Check sheet for the drawn part. Datum: minimum x, y, z corner. Units: mm. A direction names the side the tool comes from. Give positions to 0.01 mm unless a question says otherwise; leave off trailing zeros. Order: outer loops, then holes, each group sorted by start corner. A loop starts at its lowest first (then second) coordinate and runs counter-clockwise, first axis right, second up.
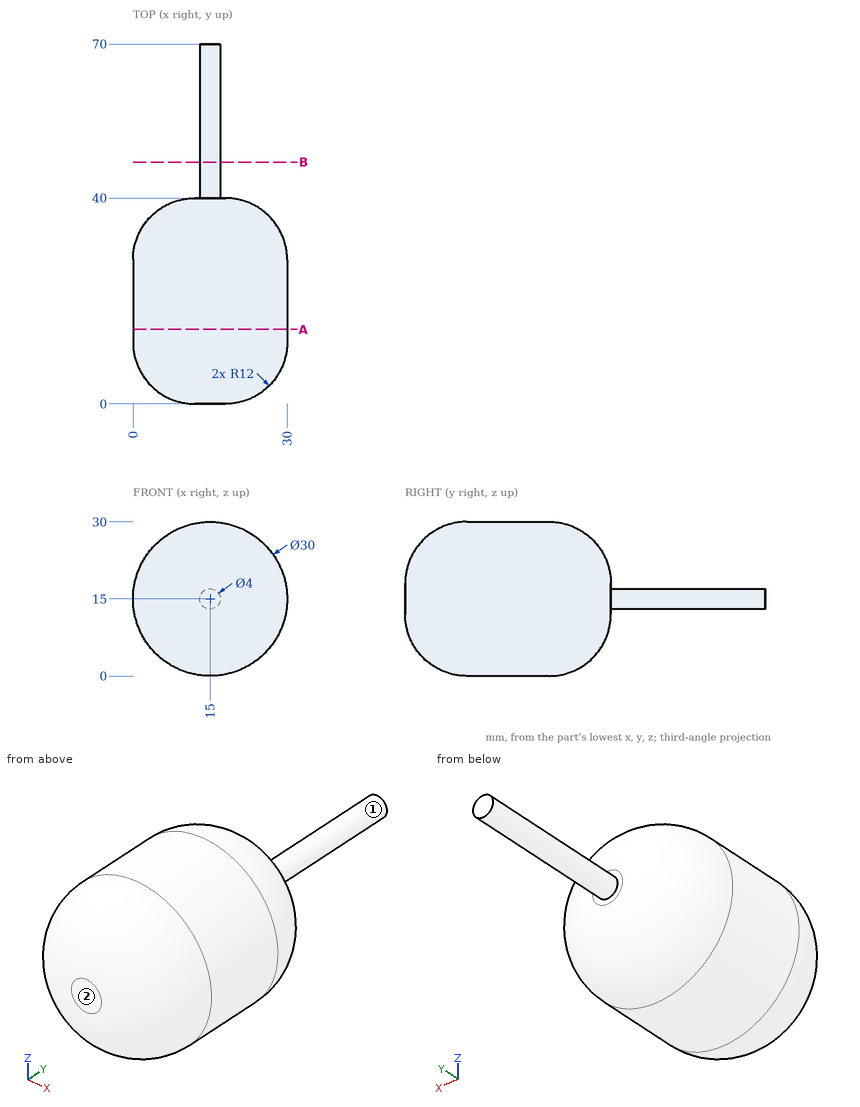
(1) Set-up check for the marked faces 1 and 2: record each of +Z, -Z, +X, -X, +Y, -Y from which the full face is reachable in a straight line by a thin tool's end or side.
Solved:
face 1: +Y
face 2: +Z, -Z, +X, -X, -Y
(2) Section check A-A, the plane y = 14.5. Enter the section's corners in (x, z), then the cut area to 3 significant figures.
Solved:
outline: circle Ø30 at (15, 15)
area: 707 mm2
(3) Scan lines: line 1 (X direction, y = 24, z = 7); line 2 (Y direction, x = 4.5, z = 7.5); line 3 (Z direction, x = 23, y = 6). Record each from-to range of solid material in increasing order.
Solved:
line 1: x = 2.31 to 27.69
line 2: y = 5.22 to 34.78
line 3: z = 4.26 to 25.74
(4) Go/stop test with flat-tipped pins: pin 1 (12 mm diameter, centred on x = 15.5, y = 11.5, fed in from -Z); pin 2 (2 mm diameter, centred on x = 13, y = 56, fed in from -Z); pin 3 (2 mm diameter, centred on x = 23, z = 19.5, fed in from +Y) (3 decimals); pin 4 (4 mm diameter, centred on x = 19.5, z = 16, fed in from +Y). Record where each tip stops, or that it passes through.
Solved:
pin 1: stops at z = 0
pin 2: stops at z = 13.27
pin 3: stops at y = 38.825
pin 4: stops at y = 40
(5) Section check B-B, the plane y = 47. Enter the section's corners in (x, z).
Solved:
outline: circle Ø4 at (15, 15)
